from build123d import *

# Parameters (mm, degrees)
BOSS_EXTRUDE1_DEPTH                             = 45
SKETCH3_R                                       = 13.7
CUT_EXTRUDE1_DEPTH                              = 3
CSK_FOR_M2_FLAT_HEAD_MACHINE_SCREW1_D           = 2.4
CSK_FOR_M2_FLAT_HEAD_MACHINE_SCREW1_CSINK_D     = 4.4
CSK_FOR_M2_FLAT_HEAD_MACHINE_SCREW1_CSINK_ANGLE = 90
SKETCH10_R                                      = 7.25
CUT_EXTRUDE2_DEPTH                              = 69.23672032
SKETCH15_R                                      = 48.495489481
SKETCH15_R_2                                    = 44
CUT_EXTRUDE4_DEPTH                              = 70.822990483
SKETCH11_R                                      = 10.5
CUT_EXTRUDE3_DEPTH                              = 2
CBORE_FOR_M5_HEX_HEAD_BOLT1_D                   = 3.4
CBORE_FOR_M5_HEX_HEAD_BOLT1_CBORE_D             = 5.3
CBORE_FOR_M5_HEX_HEAD_BOLT1_CBORE_DEPTH         = 4
SKETCH19_W                                      = 66.35
SKETCH19_H                                      = 3.175
BOSS_EXTRUDE5_DEPTH                             = 53.175
BOSS_EXTRUDE9_DEPTH                             = 8
FILLET2_R                                       = 8
FILLET3_R                                       = 8
SKETCH24_W                                      = 3.175
SKETCH24_H                                      = 11
BOSS_EXTRUDE10_DEPTH                            = 5.175
SKETCH25_W                                      = 3.175
SKETCH25_H                                      = 11
BOSS_EXTRUDE11_DEPTH                            = 60
FILLET4_R                                       = 2


with BuildPart() as part:
    # Sketch1 → Boss-Extrude1 (new body)
    with BuildSketch(Plane.XY):
        Polygon((-37.5, 0), (-27.038942926, 0), (-15, 32), (15, 32), (27.038942926, 0), (37.5, 0), (37.5, 5), (30.5, 5), (18.084840108, 38), (-18.084840108, 38), (-30.5, 5), (-37.5, 5), align=None)
    extrude(amount=BOSS_EXTRUDE1_DEPTH)

    # Sketch3 → Cut-Extrude1 (cut)
    with BuildSketch(Plane(origin=(0, 38, 0), x_dir=(1, 0, 0), z_dir=(0, 1, 0))):
        with Locations(Location((0, -30, 0), (0, 0, 180))):
            Circle(SKETCH3_R)
    extrude(amount=-CUT_EXTRUDE1_DEPTH, mode=Mode.SUBTRACT)

    # CSK for M2 Flat Head Machine Screw1 (through all)
    with Locations(Plane(origin=(0, 32, 0), x_dir=(-1, 0, 0), z_dir=(0, -1, 0))):
        with Locations((12, -42), (-12, -42), (-12, -18), (12, -18)):
            CounterSinkHole(CSK_FOR_M2_FLAT_HEAD_MACHINE_SCREW1_D / 2, CSK_FOR_M2_FLAT_HEAD_MACHINE_SCREW1_CSINK_D / 2, counter_sink_angle=CSK_FOR_M2_FLAT_HEAD_MACHINE_SCREW1_CSINK_ANGLE)

    # Sketch10 → Cut-Extrude2 (cut, through all)
    with BuildSketch(Plane(origin=(0, 35, 0), x_dir=(1, 0, 0), z_dir=(0, 1, 0))):
        with Locations(Location((0, -30, 0), (0, 0, 180))):
            Circle(SKETCH10_R)
    extrude(amount=-CUT_EXTRUDE2_DEPTH, mode=Mode.SUBTRACT)

    # Sketch15 → Cut-Extrude4 (cut, through all)
    with BuildSketch(Plane(origin=(0, 38, 0), x_dir=(1, 0, 0), z_dir=(0, 1, 0))):
        with Locations((0, -14.25)):
            Circle(SKETCH15_R)
        with Locations((0, -14.25)):
            Circle(SKETCH15_R_2, mode=Mode.SUBTRACT)
    extrude(amount=-CUT_EXTRUDE4_DEPTH, mode=Mode.SUBTRACT)

    # Sketch11 → Cut-Extrude3 (cut)
    with BuildSketch(Plane.XZ.offset(-32)):
        with Locations((0, 30)):
            Circle(SKETCH11_R)
    extrude(amount=-CUT_EXTRUDE3_DEPTH, mode=Mode.SUBTRACT)

    # CBORE for M5 Hex Head Bolt1 (through all)
    with Locations(Plane(origin=(0, 5, 0), x_dir=(-1, 0, 0), z_dir=(0, 1, 0))):
        with Locations((34, 35.5), (34, 3.5), (-34, 3.5), (-34, 35.5)):
            CounterBoreHole(CBORE_FOR_M5_HEX_HEAD_BOLT1_D / 2, CBORE_FOR_M5_HEX_HEAD_BOLT1_CBORE_D / 2, CBORE_FOR_M5_HEX_HEAD_BOLT1_CBORE_DEPTH)

    # Sketch19 → Boss-Extrude5 (add)
    with BuildSketch(Plane(origin=(0, 38, 0), x_dir=(1, 0, 0), z_dir=(0, 1, 0))):
        with Locations((0, -11.5875)):
            Rectangle(SKETCH19_W, SKETCH19_H)
    extrude(amount=BOSS_EXTRUDE5_DEPTH)

    # Sketch23 → Boss-Extrude9 (add)
    with BuildSketch(Plane(origin=(0, 0, 10), x_dir=(-1, 0, 0), z_dir=(0, 0, -1))):
        Polygon((-33.175, 38), (-30, 38), (-30, 88), (33.175, 88), (33.175, 91.175), (-33.175, 91.175), align=None)
    extrude(amount=BOSS_EXTRUDE9_DEPTH)

    # Fillet2
    fillet2_edges = [part.edges().sort_by_distance(p)[0] for p in [
        (18.084840108, 38, 11.5875),
    ]]
    fillet(fillet2_edges, radius=FILLET2_R)

    # Fillet3
    fillet3_edges = [part.edges().sort_by_distance(p)[0] for p in [
        (-18.084840108, 38, 11.5875),
    ]]
    fillet(fillet3_edges, radius=FILLET3_R)

    # Sketch24 → Boss-Extrude10 (add)
    with BuildSketch(Plane(origin=(0, 0, 2), x_dir=(-1, 0, 0), z_dir=(0, 0, -1))):
        with Locations((-31.5875, 70.5)):
            Rectangle(SKETCH24_W, SKETCH24_H)
    extrude(amount=BOSS_EXTRUDE10_DEPTH)

    # Sketch25 → Boss-Extrude11 (add)
    with BuildSketch(Plane.ZY.offset(-30)):
        with Locations((-1.5875, 70.5)):
            Rectangle(SKETCH25_W, SKETCH25_H)
    extrude(amount=BOSS_EXTRUDE11_DEPTH)

    # Fillet4
    fillet4_edges = [part.edges().sort_by_distance(p)[0] for p in [
        (31.5875, 76, 2),
        (31.5875, 65, 2),
    ]]
    fillet(fillet4_edges, radius=FILLET4_R)


solid = part.part
Geometry check sheet. Reference: the model listing, model coordinates, mm. A direction names the side the tool comes from. Give positions to 0.01 mm unless a question says otherwise; leave off trailing zeros. Loops run counter-clockwise (first coordinate to the right, second up) from the corner with the lowest first, then second, coordinate; pieces in that order, holes last. Notation, with made-up numbers: (18, -29.5) -> (66, -29.5) arc R35 ccw to (66, 6.5) -> close; hole circle Ø9 at (44, 3). An arc over 180 degrees is marked (long way). Answer in a Markdown table with one row per item. Add a question column.
1) Cross-section at C-C on z = 30. Record the boundary of the cut face in (x, y), and give its area (3 significant figures).
2) Cross-section at B-B on x = 0. Record the boundary of the cut face in (y, z) (3 decimals).
3) Set-up check for faces 5 (the face through (-21.104, 15.776, 22.185)), 6 (the face through (0, 38, 5)), 7 (the face through (35.953, 3.028, 37.291)), 8 (the face through (-31, 38, 12)), 9 (the face through (2.2, 34, 37.1)): record each of +Z, -Z, +X, -X, +Y, -Y from which the full face is reachable in a straight line by a thin tool's end or side.
4) Cross-section at A-A on z = 3.5. State how many separate pieces and enclosed holes the cut face has, and give its area (3 significant figures).
5) Material ranges on probe 1 along Y at (x, z) = (-5, 8.5) (3 decimals); probe 2 along Z at (x, y) = (-34, 0.6); probe 3 along Z at (x, y) = (-24.5, 68.5) (3 decimals), recorded low to high. Write a range as from..to.
6) Draft check along Y on faces 1 (the face through (31, 38, 8)), 2 (the face through (-1, 88, 6)), 3 (the face through (-37.5, 3, 18)), 4 (the face through (0, 91.175, 8)). Enter one of: pulls with the +Y half, pulls with the -Y half, needs draft (parallel to the pull), parting line crosses it, or undercut.
7) Gauge pin test, flat ends, axial feed: P1, Ø10, axis at x = 9, z = 36.5, coming from the -Y side; P2, Ø10.5, axis at x = -10.5, y = 83, coming from the -Z side; P3, Ø6, axis at x = -14, y = 28.5, coming from the -Z side; P4, Ø8, axis at y = 42.5, z = 37.5, coming from the -X side. Record the tip position at first contact, or that the pin passes through.
Outcome:
| question | item | result |
|---|---|---|
| 1 | outline | (-37.5, 0) -> (-27.04, 0) -> (-15, 32) -> (-10.5, 32) -> (-10.5, 34) -> (-7.25, 34) -> (-7.25, 35) -> (-13.7, 35) -> (-13.7, 38) -> (-18.08, 38) -> (-30.5, 5) -> (-37.5, 5) -> close; (7.25, 34) -> (10.5, 34) -> (10.5, 32) -> (15, 32) -> (27.04, 0) -> (37.5, 0) -> (37.5, 5) -> (30.5, 5) -> (18.08, 38) -> (13.7, 38) -> (13.7, 35) -> (7.25, 35) -> close |
| 1 | area | 494 mm^2 |
| 2 | outline | (32, 0) -> (38, 0) -> (38, 10) -> (88, 10) -> (88, 2) -> (91.175, 2) -> (91.175, 13.175) -> (38, 13.175) -> (38, 16.3) -> (35, 16.3) -> (35, 22.75) -> (34, 22.75) -> (34, 19.5) -> (32, 19.5) -> close; (32, 40.5) -> (34, 40.5) -> (34, 37.25) -> (35, 37.25) -> (35, 43.7) -> (38, 43.7) -> (38, 45) -> (32, 45) -> close; (65, -3.175) -> (76, -3.175) -> (76, 0) -> (65, 0) -> close |
| 3 | face 5 | +Z, -Z, -Y |
| 3 | face 6 | -Z, -X |
| 3 | face 7 | +Y |
| 3 | face 8 | +Z, -Z, -X |
| 3 | face 9 | -Y |
| 4 | separate pieces | 4 |
| 4 | enclosed holes | 0 |
| 4 | area | 953 mm^2 |
| 5 | probe 1 | y = 32..38, 88..91.175 |
| 5 | probe 2 | z = 0..1.8, 5.2..33.8, 37.2..42.18 |
| 5 | probe 3 | z = -3.175..0, 10..13.175 |
| 6 | face 1 | undercut |
| 6 | face 2 | undercut |
| 6 | face 3 | needs draft |
| 6 | face 4 | pulls with the +Y half |
| 7 | P1 | stops at y = 32 |
| 7 | P2 | stops at z = 2 |
| 7 | P3 | stops at z = 0 |
| 7 | P4 | passes through |
